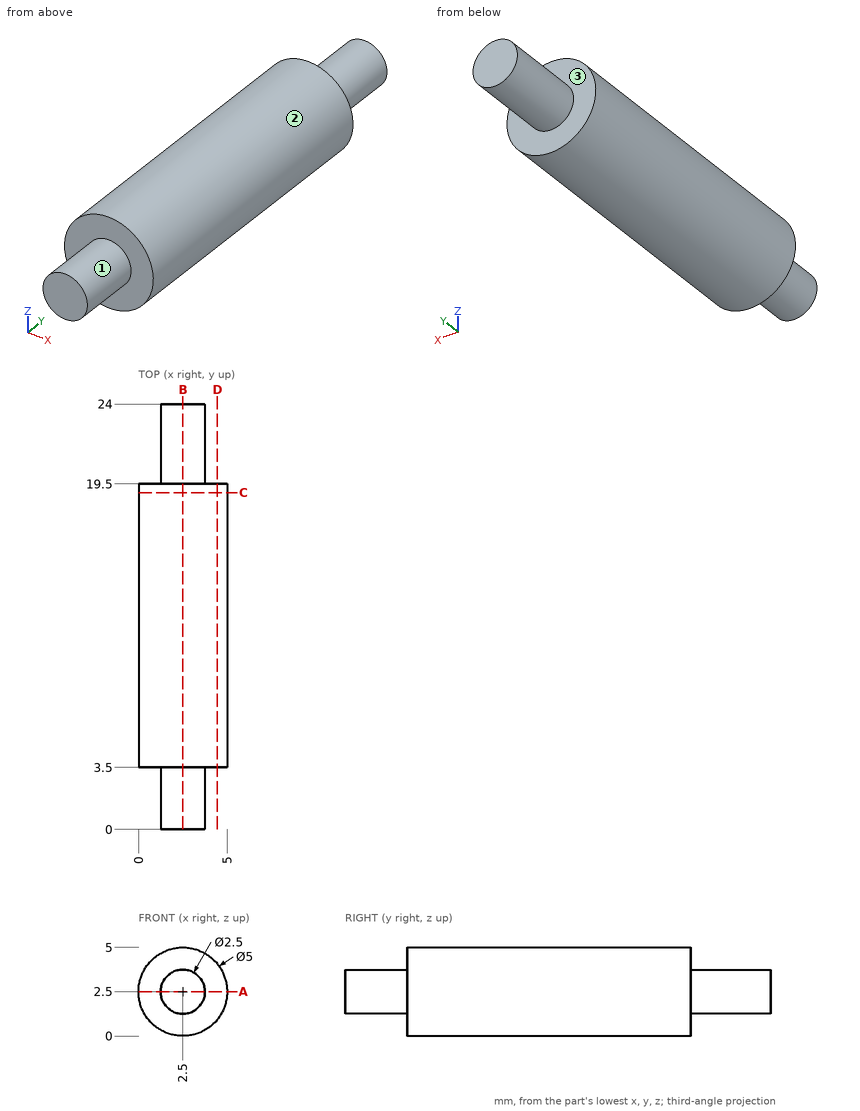
Source: three-view drawing plus pictorial views. Frame: mm from the lowest corner of the part. A direction names the side the tool comes from. Round coordinates to 2 decimals unless told otherwise and drop trailing zeros. Loops run counter-clockwise (first coordinate to the right, second up) from the corner with the lowest first, then second, coordinate; pieces in that order, holes last.
Q1. Section B-B, the plane x = 2.5. Return loops of the section in (y, z), plus the area to 3 significant figures.
Q2. Section A-A, the plane z = 2.5. Return loops of the section in (x, y).
Q3. Section D-D, the plane x = 4.45. Return loops of the section in (y, z).
Q4. Access query for the marked faces 1, 2 and 3. Directions: +Z, -Z, +X, -X, +Y, -Y. A direction counts if a zero-diameter tool reaches every point of the face in a straight line with its end or side. Return the directions, or none.
Q5. First-contact query: P1, Ø1.5, axis at y = 13, z = 4, coming from the -X side. Flat tip, straight axial feed; report the tip coordinate or a pass-through.
Q6. Ray query, line 1 (Y direction, x = 2.7, z = 4.45); line 2 (Z direction, x = 3.3, y = 3.25); line 3 (Z direction, x = 2, y = 20.5). Return the intervals inside material, ascending.
Q7. Section C-C, the plane y = 19. Return loops of the section in (x, z), plus the area to 3 significant figures.
Solutions:
1. outline: (0, 1.25) - (3.5, 1.25) - (3.5, 0) - (19.5, 0) - (19.5, 1.25) - (24, 1.25) - (24, 3.75) - (19.5, 3.75) - (19.5, 5) - (3.5, 5) - (3.5, 3.75) - (0, 3.75) - close
1. area: 100 mm2
2. outline: (0, 3.5) - (1.25, 3.5) - (1.25, 0) - (3.75, 0) - (3.75, 3.5) - (5, 3.5) - (5, 19.5) - (3.75, 19.5) - (3.75, 24) - (1.25, 24) - (1.25, 19.5) - (0, 19.5) - close
3. outline: (3.5, 0.94) - (19.5, 0.94) - (19.5, 4.06) - (3.5, 4.06) - close
4. face 1: -Y
4. face 2: +Y, -Y
4. face 3: +Y
5. P1: stops at x = 0.12
6. line 1: y = 3.5 to 19.5
6. line 2: z = 1.54 to 3.46
6. line 3: z = 1.35 to 3.65
7. outline: circle Ø5 at (2.5, 2.5)
7. area: 19.6 mm2
